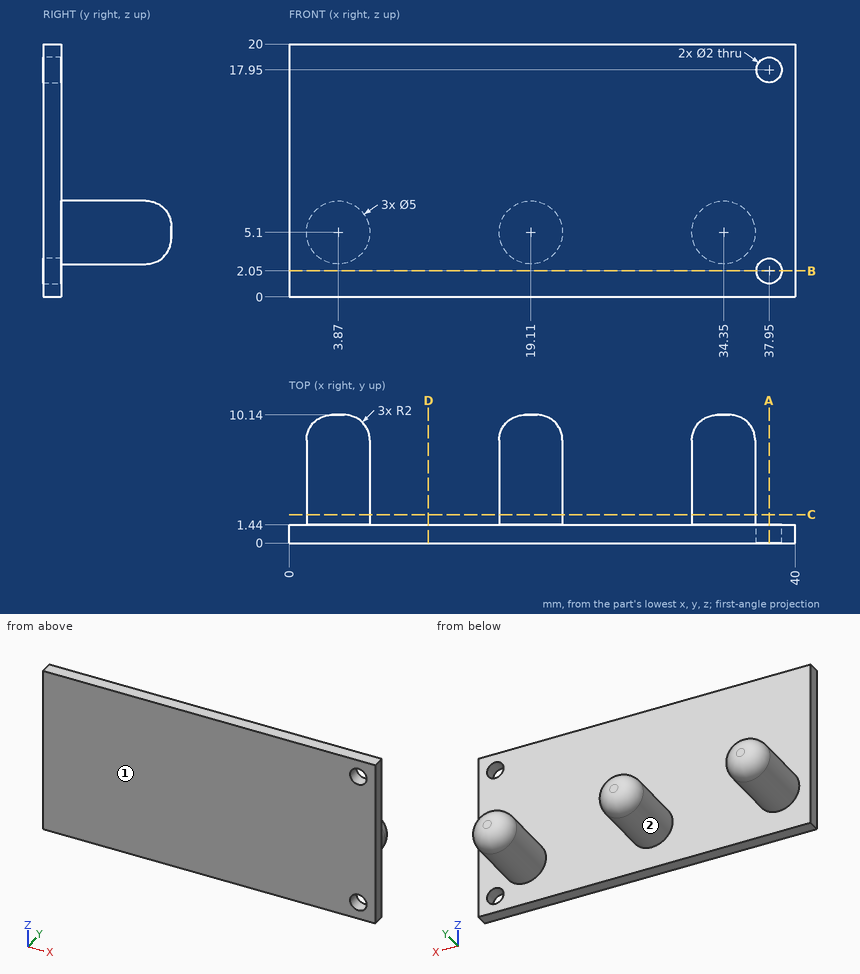
Here's the drawing with two shaded views (mm, measured from the low corner). I have some questions. Round coordinates to 2 decimals unless told otherwise and drop trailing zeros. Loops run counter-clockwise (first coordinate to the right, second up) from the corner with the lowest first, then second, coordinate; pieces in that order, holes last. Notation, with made-up numbers: M 14.25,73.25 L 72.25,73.25 A12 ccw 72.25,78.25 Z; hole C -2,-16.5 d10. An arc over 180 degrees is marked long. Answer as CSV lines item,"result".
1) For pin 1 Ø1.5 at (x, z) = (21.5, 14) entering from +Y; pin 2 Ø4 at (x, y) = (32, 8.5) entering from -Z; pin 3 Ø1.6 at (x, z) = (37.95, 17.95) entering from +Y, each with a flat end and sliding along its axis, tell me the tip position at first contact or that it passes through.
From the geometry:
pin 1,"y = 1.44"
pin 2,"z = 2.63"
pin 3,"through"
2) Imagine slicing it at D-D on x = 11. List the corners of the cut face in (y, z) for me, and give its area (3 significant figures).
From the geometry:
outline,"M 0,0 L 1.44,0 L 1.44,20 L 0,20 Z"
area,"28.8 mm^2"
3) If I drill on probe 1 along Z at (x, y) = (37.95, 0.9); probe 2 along X at (y, z) = (0.65, 17.95); probe 3 along X at (y, z) = (9, 3.5), over which ranges is the centre line in solid material (lowest first)?
From the geometry:
probe 1,"0 to 1.05, 3.05 to 16.95, 18.95 to 20"
probe 2,"0 to 36.95, 38.95 to 40"
probe 3,"2.21 to 5.53, 17.45 to 20.77, 32.69 to 36.01"
4) We'd pull the mould along X, two halves only. Please class the marked faces 1 and 2: released by +X, released by -X, zero draft, split by the parting line, or undercut.
From the geometry:
face 1,"zero draft"
face 2,"undercut"
5) Imagine slicing it at A-A on x = 37.95. List the corners of the cut face in (y, z) for me.
From the geometry:
outline,"M 0,0 L 1.44,0 L 1.44,1.05 L 0,1.05 Z; M 0,3.05 L 1.44,3.05 L 1.44,16.95 L 0,16.95 Z; M 0,18.95 L 1.44,18.95 L 1.44,20 L 0,20 Z"
6) Imagine slicing it at B-B on z = 2.05. List the corners of the cut face in (x, y) for me.
From the geometry:
outline,"M 0,0 L 36.95,0 L 36.95,1.44 L 0,1.44 Z; M 38.95,0 L 40,0 L 40,1.44 L 38.95,1.44 Z"
7) Imagine slicing it at C-C on y = 2.25. List the corners of the cut face in (x, z) for me, and give its area (3 significant figures).
From the geometry:
outline,"C 3.87,5.1 d5; C 19.11,5.1 d5; C 34.35,5.1 d5"
area,"58.9 mm^2"
